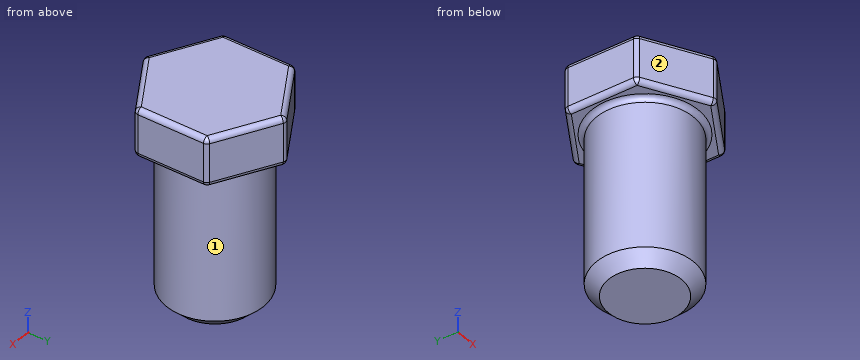
```python
from build123d import *

# Parameters (mm, degrees)
SKETCH1_R           = 2
BOSS_EXTRUDE1_DEPTH = 3.35
BOSS_EXTRUDE2_DEPTH = 2
FILLET1_R           = 0.2
FILLET2_R           = 0.2
CHAMFER1_SIZE       = 0.5


with BuildPart() as part:
    # Sketch1 → Boss-Extrude1 (new body, symmetric)
    with BuildSketch(Plane.XY):
        Circle(SKETCH1_R)
    extrude(amount=BOSS_EXTRUDE1_DEPTH, both=True)

    # Sketch2 → Boss-Extrude2 (add)
    with BuildSketch(Plane.XY.offset(3.35)):
        Polygon((0, -2.886751346), (2.5, -1.443375673), (2.5, 1.443375673), (0, 2.886751346), (-2.5, 1.443375673), (-2.5, -1.443375673), align=None)
    extrude(amount=BOSS_EXTRUDE2_DEPTH)

    # Fillet1
    fillet1_edges = [part.edges().sort_by_distance(p)[0] for p in [
        (-2, 0, 3.35),
        (-1.25, -2.165063509, 3.35),
        (1.25, -2.165063509, 3.35),
        (2.5, 0, 3.35),
        (1.25, 2.165063509, 3.35),
        (-1.25, 2.165063509, 3.35),
        (-2.5, 0, 3.35),
        (-1.25, -2.165063509, 5.35),
        (1.25, -2.165063509, 5.35),
        (2.5, 0, 5.35),
        (1.25, 2.165063509, 5.35),
        (-1.25, 2.165063509, 5.35),
        (-2.5, 0, 5.35),
    ]]
    fillet(fillet1_edges, radius=FILLET1_R)

    # Fillet2
    fillet2_edges = [part.edges().sort_by_distance(p)[0] for p in [
        (-2.5, -1.443375673, 4.35),
        (-2.5, 1.443375673, 4.35),
        (0, 2.886751346, 4.35),
        (2.5, 1.443375673, 4.35),
        (2.5, -1.443375673, 4.35),
        (0, -2.886751346, 4.35),
        (2.436285816, 1.406590271, 5.29637683),
        (2.436285816, -1.406590271, 5.29637683),
        (0, 2.813180543, 5.29637683),
        (0, -2.813180543, 5.29637683),
        (-2.436285816, 1.406590271, 5.29637683),
        (-2.436285816, -1.406590271, 5.29637683),
        (-2.436285816, 1.406590271, 3.40362317),
        (0, 2.813180543, 3.40362317),
        (-2.436285816, -1.406590271, 3.40362317),
        (2.436285816, 1.406590271, 3.40362317),
        (0, -2.813180543, 3.40362317),
        (2.436285816, -1.406590271, 3.40362317),
    ]]
    fillet(fillet2_edges, radius=FILLET2_R)

    # Chamfer1
    chamfer1_edges = [part.edges().sort_by_distance(p)[0] for p in [
        (-2, 0, -3.35),
    ]]
    chamfer(chamfer1_edges, length=CHAMFER1_SIZE)


solid = part.part
```
Geometry check sheet. Reference: the model listing, model coordinates, mm. Face numbers are marked on the shaded views. A direction names the side the tool comes from. Give positions to 0.01 mm unless a question says otherwise; leave off trailing zeros. Loops run counter-clockwise (first coordinate to the right, second up) from the corner with the lowest first, then second, coordinate; pieces in that order, holes last. Notation, with made-up numbers: (-17.75, 78.5) - (39.25, 78.5) arc R22 cw to (39.25, 108.5) - close; hole circle Ø8 at (-9.75, 26.25). An arc over 180 degrees is marked (long way). Use CSV: the item, a comma, the result in double quotes. Start each with the question number.
Q1. Section check B-B, the plane z = -1.75. Record the cut outline in (x, y), and give its area (3 significant figures).
Q2. Scan lines: probe 1 along X at (y, z) = (0.1, -2.5); probe 2 along Y at (x, z) = (-0.55, 3.25); probe 3 along Y at (x, z) = (-1.65, 2.5). Record each from-to range of solid material in increasing order. Write a range as from..to.
Q3. Access from +Z, -Z, +X, -X, +Y, -Y to the whole of each face (thin tool, end or side, straight path). Record for the marked faces 1 and 2.
Q4. Go/stop test with a flat-tipped pin: pin 1 Ø3 at (x, z) = (0.5, -0.5) entering from -Y. Record where the tip stops, or that it passes through.
Q5. Section check A-A, the plane y = 0. Record the cut outline in (x, z).
Findings below:
1,outline,"circle Ø4 at (0, 0)"
1,area,"12.6 mm^2"
2,probe 1,"x = -2..2"
2,probe 2,"y = -1.95..1.95"
2,probe 3,"y = -1.13..1.13"
3,face 1,"-Z"
3,face 2,"+Z, -Z, -X, -Y"
4,pin 1,"stops at y = -2"
5,outline,"(-2.5, 3.55) arc R0.2 ccw to (-2.3, 3.35) - (-2.2, 3.35) arc R0.2 cw to (-2, 3.15) - (-2, -2.85) - (-1.5, -3.35) - (1.5, -3.35) - (2, -2.85) - (2, 3.15) arc R0.2 cw to (2.2, 3.35) - (2.3, 3.35) arc R0.2 ccw to (2.5, 3.55) - (2.5, 5.15) arc R0.2 ccw to (2.3, 5.35) - (-2.3, 5.35) arc R0.2 ccw to (-2.5, 5.15) - close"
